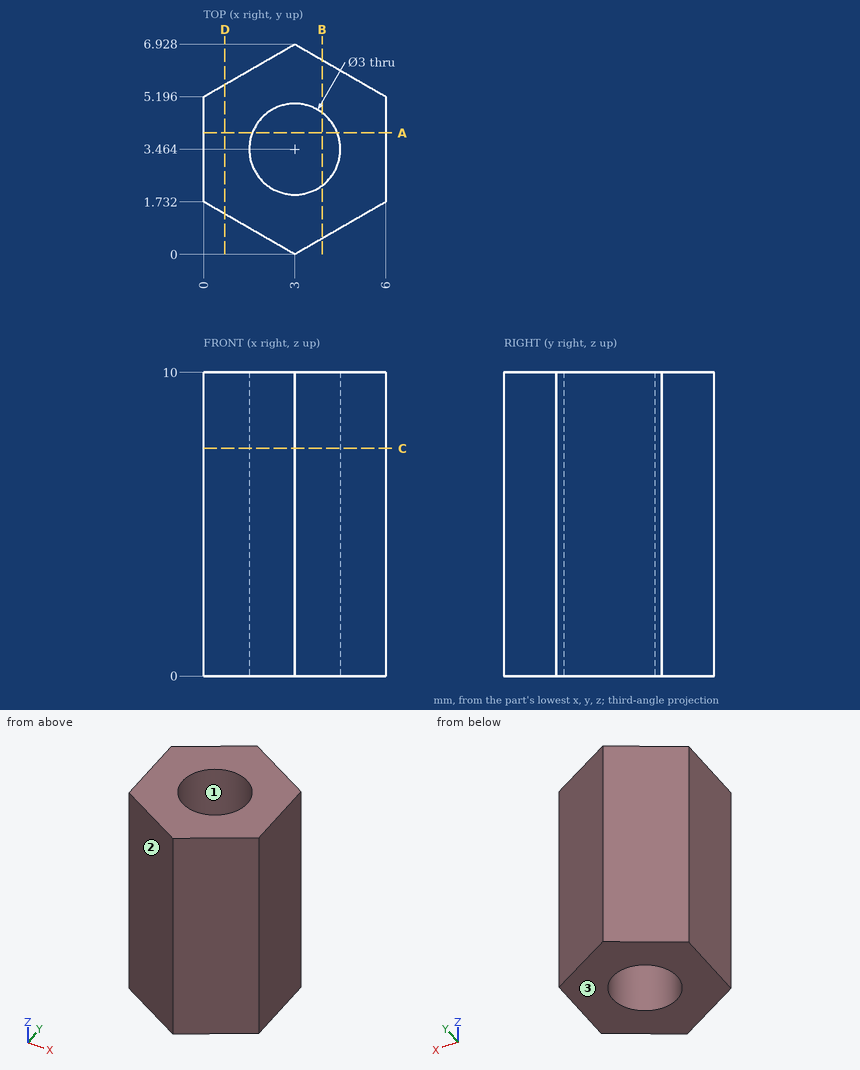
Check sheet for the drawn part. Datum: minimum x, y, z corner. Units: mm. Give positions to 0.01 mm unless a question says otherwise; leave off trailing zeros. Loops run counter-clockwise (first coordinate to the right, second up) from the corner with the lowest first, then second, coordinate; pieces in that order, holes last. Notation, with made-up numbers: M 86,34.25 L 93,34.25 A26 ccw 93,60.25 Z; hole C 11,-10 d8. An arc over 180 degrees is marked long. Answer as CSV lines item,"result".
Item 1: Sectioned sample at D-D, the plane x = 0.7. Enter the section's corners in (y, z).
Reply:
outline,"M 1.33,0 L 5.6,0 L 5.6,10 L 1.33,10 Z"
Item 2: Scan lines: L1, parallel to X at y = 4.5, z = 6.5 (1 decimal); L2, parallel to Y at x = 1.9, z = 5.25 (1 decimal); L3, parallel to X at y = 2.25, z = 1.75. Record each from-to range of solid material in increasing order.
Reply:
L1,"0 to 1.9, 4.1 to 6"
L2,"0.6 to 2.4, 4.5 to 6.3"
L3,"0 to 2.12, 3.88 to 6"
Item 3: Sectioned sample at B-B, the plane x = 3.9. Enter the section's corners in (y, z).
Reply:
outline,"M 0.52,0 L 2.26,0 L 2.26,10 L 0.52,10 Z; M 4.66,0 L 6.41,0 L 6.41,10 L 4.66,10 Z"
Item 4: Draft check along Y on the marked faces 1, 2 and 3. Enter one of: pulls with the +Y half, pulls with the -Y half, needs draft (parallel to the pull), parting line crosses it, or undercut.
Reply:
face 1,"undercut"
face 2,"pulls with the -Y half"
face 3,"needs draft"
Item 5: Sectioned sample at A-A, the plane y = 4. Enter the section's corners in (x, z), then the cut area to 3 significant figures.
Reply:
outline,"M 0,0 L 1.6,0 L 1.6,10 L 0,10 Z; M 4.4,0 L 6,0 L 6,10 L 4.4,10 Z"
area,"32.0 mm^2"
Item 6: Depth check by flat-ended pin: pin 1 Ø3 at (x, z) = (1, 6.5) entering from -Y. Enter the tip coordinate at first touch or a pass-through.
Reply:
pin 1,"y = 0.29"
Item 7: Sectioned sample at C-C, the plane z = 7.5. Enter the section's corners in (x, y).
Reply:
outline,"M 0,1.73 L 3,0 L 6,1.73 L 6,5.2 L 3,6.93 L 0,5.2 Z; hole C 3,3.46 d3"
